Here's how the part is built. I have some questions about the finished solid (model axes, mm). A direction names the side the tool comes from. Coordinates: 2 decimals unless noted, no trailing zeros. Write each loop counter-clockwise with the first axis right and the second up, starting at its lowest first coordinate (ties: lowest second). Pieces come first, ordered by that corner, then holes. Notation, with made-up numbers: (-3.5, 75.25) - (44.5, 75.25) arc R22 cw to (44.5, 109.25) - close; hole circle Ø4 at (-29.5, -7). An arc over 180 degrees is marked (long way). Answer in a Markdown table with one row per item. Add a question column.
Item 1: If I drill on probe 1 along Y at (x, z) = (20, 0.6); probe 2 along X at (y, z) = (25, 6.5); probe 3 along Z at (x, y) = (39.4, 0), over which ranges is the centre line in solid material (lowest first)? Write a range as from..to.
Item 2: We'd pull the mould along X, two halves only. Please class faces 4 (the face through (18.7, -8.94, 0.49)), 5 (the face through (-39.43, -39.4, 6.16)), 6 (the face through (39.43, 39.4, 6.16)): +X half, -X half, draft (parallel to the pull), parting line (faces both ways), or undercut.
Item 3: Imagine slicing it at B-B (y = 9). Please give me the cut outline in (x, z).
Item 4: Imagine slicing it at D-D (z = 2.75). Please give me the cut outline in (x, y).
Item 5: Imagine slicing it at C-C (z = 7). Please give me the cut outline in (x, y), plus the area to 3 significant figures.
Item 6: I'm going to push a flat-ended pin straight in: pin 1 (22.5 mm diameter, centred on x = -6, y = 12, fed in from +Z). Where does the tip first touch, or does it pass through?
Item 7: Imagine slicing it at A-A (x = 20). Please give me the cut outline in (y, z).
Item 8: Which directions (+Z, -Z, +X, -X, +Y, -Y) give clear straight access to the entire face, cutting with the end or side of a thin tool? Please do faces 1 (the face through (39, 0, 9)), 2 (the face through (39.4, -39.43, 6.16)), 3 (the face through (-1, 1, 1)).
from build123d import *

# Parameters (mm, degrees)
CYLINDER001_R     = 2
CYLINDER001_DEPTH = 10
SKETCH005_W       = 75
SKETCH005_H       = 75
SKETCH005_R       = 1.3
EXTRUDE005_DEPTH  = 1
SKETCH004_W       = 75
SKETCH004_H       = 75
EXTRUDE004_DEPTH  = 12.5


with BuildPart() as obj1:
    # Cylinder001 → Cylinder001 (new body)
    with BuildSketch(Plane(origin=(35, 0, 7), x_dir=(0, 0, -1), z_dir=(1, 0, 0))):
        Circle(CYLINDER001_R)
    extrude(amount=CYLINDER001_DEPTH)


with BuildPart() as solar_rahmen_boden:
    # Sketch005 → Extrude005 (new body)
    with BuildSketch(Plane.XY):
        Rectangle(SKETCH005_W, SKETCH005_H)
        with Locations((20, 9)):
            Circle(SKETCH005_R, mode=Mode.SUBTRACT)
        with Locations((20, -9)):
            Circle(SKETCH005_R, mode=Mode.SUBTRACT)
    extrude(amount=EXTRUDE005_DEPTH)


with BuildPart() as obj2:
    # Sketch004 → Extrude004 (new body)
    with BuildSketch(Plane.XY):
        with BuildLine():
            Line((-38, 40), (38, 40))
            ThreePointArc((40, 38), (39.414214, 39.414214), (38, 40))
            Line((40, 38), (40, -38))
            ThreePointArc((38, -40), (39.414214, -39.414214), (40, -38))
            Line((38, -40), (-38, -40))
            ThreePointArc((-40, -38), (-39.414214, -39.414214), (-38, -40))
            Line((-40, -38), (-40, 38))
            ThreePointArc((-38, 40), (-39.414214, 39.414214), (-40, 38))
        make_face()
        Rectangle(SKETCH004_W, SKETCH004_H, mode=Mode.SUBTRACT)
    extrude(amount=EXTRUDE004_DEPTH)

    # Fusion002: union solar_rahmen_boden
    add(solar_rahmen_boden.part)

    # Cut001: cut obj1
    add(obj1.part, mode=Mode.SUBTRACT)


solid = obj2.part
Here are the results:
| question | item | result |
|---|---|---|
| 1 | probe 1 | y = -40..-10.3, -7.7..7.7, 10.3..40 |
| 1 | probe 2 | x = -40..-37.5, 37.5..40 |
| 1 | probe 3 | z = 0..5, 9..12.5 |
| 2 | face 4 | undercut |
| 2 | face 5 | -X half |
| 2 | face 6 | +X half |
| 3 | outline | (-40, 0) - (18.7, 0) - (18.7, 1) - (-37.5, 1) - (-37.5, 12.5) - (-40, 12.5) - close; (21.3, 0) - (40, 0) - (40, 12.5) - (37.5, 12.5) - (37.5, 1) - (21.3, 1) - close |
| 4 | outline | (-40, -38) arc R2 ccw to (-38, -40) - (38, -40) arc R2 ccw to (40, -38) - (40, 38) arc R2 ccw to (38, 40) - (-38, 40) arc R2 ccw to (-40, 38) - close; hole (-37.5, -37.5) - (37.5, -37.5) - (37.5, 37.5) - (-37.5, 37.5) - close |
| 5 | outline | (-40, -38) arc R2 ccw to (-38, -40) - (38, -40) arc R2 ccw to (40, -38) - (40, -2) - (37.5, -2) - (37.5, -37.5) - (-37.5, -37.5) - (-37.5, 37.5) - (37.5, 37.5) - (37.5, 2) - (40, 2) - (40, 38) arc R2 ccw to (38, 40) - (-38, 40) arc R2 ccw to (-40, 38) - close |
| 5 | area | 762 mm2 |
| 6 | pin 1 | stops at z = 1 |
| 7 | outline | (-40, 0) - (-10.3, 0) - (-10.3, 1) - (-37.5, 1) - (-37.5, 12.5) - (-40, 12.5) - close; (-7.7, 0) - (7.7, 0) - (7.7, 1) - (-7.7, 1) - close; (10.3, 0) - (40, 0) - (40, 12.5) - (37.5, 12.5) - (37.5, 1) - (10.3, 1) - close |
| 8 | face 1 | +X |
| 8 | face 2 | +Z, -Z, +X, -Y |
| 8 | face 3 | +Z |
